Input: part model. Units: mm. Frame: model coordinates. Give positions to 0.01 mm unless a question says otherwise; leave off trailing zeros. Loops run counter-clockwise (first coordinate to the right, second up) from the corner with the lowest first, then second, coordinate; pieces in that order, holes last. Notation, with made-up numbers: M -31.5,58.25 L -13.5,58.25 A19 ccw -13.5,65.25 Z; hole C -17,-12 d4. An arc over 180 degrees is marked long. Use CSV: the item, a comma, the result in double quotes. Start each with the question number.
Q1. Material intervals for line 1 along Z through (x, y) = (-0.1, 0.1); line 2 along Y through (x, z) = (0.2, -2.75); line 3 along Y through (x, z) = (-0.1, -5.75), sorted ascending.
Q2. Section C-C, the plane z = -6.25. Output: boundary loops of the cut face in (x, y).
Q3. Section B-B, the plane y = 0.7. Output: boundary loops of the cut face in (x, z), plus the area to 3 significant figures.
Q4. Section A-A, the plane x = -0.3. Output: boundary loops of the cut face in (y, z).
from build123d import *

# Parameters (mm, degrees)
BOSS_EXTRUDE1_DEPTH = 0.45
FILLET1_R           = 0.2


with BuildPart() as part:
    # Sketch1 → Boss-Extrude1 (new, symmetric)
    with BuildSketch(Plane(origin=(0, 0, 0), x_dir=(0, 0, -1), z_dir=(1, 0, 0))):
        Polygon((0, 0), (7.089102275, 1.25), (15, 1.25), (15, 0), align=None)
    extrude(amount=BOSS_EXTRUDE1_DEPTH, both=True)

    # Fillet1
    fillet1_edges = [part.edges().sort_by_distance(p)[0] for p in [
        (0, 0, 0),
    ]]
    fillet(fillet1_edges, radius=FILLET1_R)


solid = part.part
A:
1,line 1,"-15 to -2.11"
1,line 2,"0 to 0.48"
1,line 3,"0 to 1.01"
2,outline,"M -0.45,0 L 0.45,0 L 0.45,1.1 L -0.45,1.1 Z"
3,outline,"M -0.45,-15 L 0.45,-15 L 0.45,-3.97 L -0.45,-3.97 Z"
3,area,"9.93 mm^2"
4,outline,"M 0,-15 L 1.25,-15 L 1.25,-7.09 L 0.4,-2.25 A0.2 ccw 0,-2.29 Z"
